```python
from build123d import *

# Parameters (mm, degrees)
F0_R     = 3
F1_DEPTH = 2
F2_T     = -1
F4_W     = 4
F4_H     = 1
F4_R     = 4
F4_R_2   = 3
F5_DEPTH = 1


# Not quite as in the source:
# - a feature of the source that left no trace in its solid (it failed there, or was rolled back) is left out


with BuildPart() as f1:
    # F0 (on Top) → F1 (new body)
    with BuildSketch(Plane.XY):
        with BuildLine():
            ThreePointArc((76, 31), (0, 107), (-76, 31))
            Line((-76, 31), (-76, -31))
            Line((-76, -31), (-76, -69))
            Line((-76, -69), (-70, -69))
            Line((-70, -69), (-70, -47.9877756238))
            Line((-70, -47.9877756238), (-66, -47.9877756238))
            Line((-66, -47.9877756238), (-66, -40.0317243588))
            ThreePointArc((-66, -40.0317243588), (-61.2993566139, -29.9422610746), (-70, -23.00020646))
            Line((-70, -23.00020646), (-70, 31))
            ThreePointArc((-70, 31), (-66.3741952073, 53.2365962005), (-55.8723939833, 73.1696050559))
            ThreePointArc((-55.8723939833, 73.1696050559), (-43.5714285714, 73.6911069456), (-43.3010754044, 86.0001533527))
            ThreePointArc((-43.3010754044, 86.0001533527), (-22.9127613494, 97.1438233499), (0, 101))
            ThreePointArc((0, 101), (22.9127613494, 97.1438233499), (43.3010754044, 86.0001533527))
            ThreePointArc((43.3010754044, 86.0001533527), (43.5714285714, 73.6911069456), (55.8723939833, 73.1696050559))
            ThreePointArc((55.8723939833, 73.1696050559), (66.3741952073, 53.2365962005), (70, 31))
            Line((70, 31), (70, -23.00020646))
            ThreePointArc((70, -23.00020646), (61.2993566139, -29.9422610746), (66, -40.0317243588))
            Line((66, -40.0317243588), (66, -47.9877756238))
            Line((66, -47.9877756238), (70, -47.9877756238))
            Line((70, -47.9877756238), (70, -69))
            Line((70, -69), (76, -69))
            Line((76, -69), (76, -31))
            Line((76, -31), (76, 31))
        make_face()
        with Locations((-70.0609609485, -32)):
            Circle(F0_R, mode=Mode.SUBTRACT)
        with Locations((70.0609609485, -32)):
            Circle(F0_R, mode=Mode.SUBTRACT)
        with Locations((-50, 79.9897948557)):
            Circle(F0_R, mode=Mode.SUBTRACT)
        with Locations((50, 79.9897948557)):
            Circle(F0_R, mode=Mode.SUBTRACT)
    extrude(amount=F1_DEPTH)

    # F2
    f2_openings = [f1.faces().sort_by_distance(p)[0] for p in [
        (0, 104.674489, 2),
    ]]
    offset(amount=F2_T, openings=f2_openings, kind=Kind.INTERSECTION)

    # F4 (on face) → F5 (cut)
    with BuildSketch(Plane.XY.offset(2)):
        with Locations((73, -68.5)):
            Rectangle(F4_W, F4_H)
        with Locations((-73, -68.5)):
            Rectangle(F4_W, F4_H)
        with Locations((-70.0609609485, -32)):
            Circle(F4_R)
        with Locations((-70.0609609485, -32)):
            Circle(F4_R_2, mode=Mode.SUBTRACT)
        with Locations((70.0609609485, -32)):
            Circle(F4_R)
        with Locations((70.0609609485, -32)):
            Circle(F4_R_2, mode=Mode.SUBTRACT)
        with Locations((-50, 79.9897948557)):
            Circle(F4_R)
        with Locations((-50, 79.9897948557)):
            Circle(F4_R_2, mode=Mode.SUBTRACT)
        with Locations((50, 79.9897948557)):
            Circle(F4_R)
        with Locations((50, 79.9897948557)):
            Circle(F4_R_2, mode=Mode.SUBTRACT)
    extrude(amount=-F5_DEPTH, mode=Mode.SUBTRACT)


solid = f1.part
```
Here's how the part is built. I have some questions about the finished solid (model axes, mm). A direction names the side the tool comes from. Round coordinates to 2 decimals unless told otherwise and drop trailing zeros. Order: outer loops, then holes, each group sorted by start corner. A loop starts at its lowest first (then second) coordinate and runs counter-clockwise, first axis right, second up. Notation, with made-up numbers: (83.5, 67) -> (111.5, 67) arc R22 ccw to (111.5, 92) -> close; hole circle Ø11 at (5.5, -33.75). An arc over 180 degrees is marked (long way). Use a Markdown table: item, result. Add a question column.
(1) For pin 1 Ø9.5 at (x, y) = (50, 79.99) entering from -Z; pin 2 Ø1.1 at (x, z) = (-68, 1.5) entering from +Y; pin 3 Ø1 at (x, z) = (31, 1.5) entering from +Y, each with a flat end and sliding along its axis, tell me the tip position at first contact or that it passes through.
(2) For faces 1 (the face through (61.34, -29.78, 0.99)), 2 (the face through (67.032, 54.404, 1.493)), which set-ups out of +Z, -Z, +X, -X, +Y, -Y let a thin tool reach every point of the face, with its end or its side?
(3) If we mould it in two halves opening along X, with no side actions, what happens to faces 3 (the face through (-72.44, -33.83, 0.49)), 4 (the face through (-51, 72, 0))? For each: released by +X, released by -X, zero draft, split by the parting line, or undercut.
(4) Suppose I cut it at D-D, the plane x = -29. Please give me the cut outline in (y, z), and give its area (3 significant figures).
(5) Suppose I cut it at A-A, the plane y = -32. Please give me the cut outline in (x, z), and give its area (3 significant figures).
(6) Suppose I cut it at C-C, the plane y = -7.5. Please give me the cut outline in (x, z), and give its area (3 significant figures).
(7) Suppose I cut it at B-B, the plane x = 50. Please give me the cut outline in (y, z), and give its area (3 significant figures).
(8) I need wall thicknesses on line 1 along X through (y, z) = (-51, 1.3); line 2 along X through (y, z) = (9.5, 0.9); line 3 along Y through (x, z) = (64, 1.6). Which ranges of each line are inside material? Lowest first, please.
Verdict:
| question | item | result |
|---|---|---|
| 1 | pin 1 | z = 0 |
| 1 | pin 2 | y = 66.02 |
| 1 | pin 3 | y = 100.61 |
| 2 | face 1 | +Z, -Z |
| 2 | face 2 | +Z |
| 3 | face 3 | undercut |
| 3 | face 4 | zero draft |
| 4 | outline | (94.71, 0) -> (101.25, 0) -> (101.25, 2) -> (100.17, 2) -> (100.17, 1) -> (95.81, 1) -> (95.81, 2) -> (94.71, 2) -> close |
| 4 | area | 8.72 mm2 |
| 5 | outline | (-76, 0) -> (-73.06, 0) -> (-73.06, 1) -> (-75, 1) -> (-75, 2) -> (-76, 2) -> close; (-67.06, 0) -> (-61.06, 0) -> (-61.06, 2) -> (-62.06, 2) -> (-62.06, 1) -> (-67.06, 1) -> close; (61.06, 0) -> (67.06, 0) -> (67.06, 1) -> (62.06, 1) -> (62.06, 2) -> (61.06, 2) -> close; (73.06, 0) -> (76, 0) -> (76, 2) -> (75, 2) -> (75, 1) -> (73.06, 1) -> close |
| 5 | area | 21.9 mm2 |
| 6 | outline | (-76, 0) -> (-70, 0) -> (-70, 2) -> (-71, 2) -> (-71, 1) -> (-75, 1) -> (-75, 2) -> (-76, 2) -> close; (70, 0) -> (76, 0) -> (76, 2) -> (75, 2) -> (75, 1) -> (71, 1) -> (71, 2) -> (70, 2) -> close |
| 6 | area | 16.0 mm2 |
| 7 | outline | (70.99, 0) -> (76.99, 0) -> (76.99, 1) -> (71.99, 1) -> (71.99, 2) -> (70.99, 2) -> close; (82.99, 0) -> (88.24, 0) -> (88.24, 2) -> (86.9, 2) -> (86.9, 1) -> (82.99, 1) -> close |
| 7 | area | 13.6 mm2 |
| 8 | line 1 | -76 to -75, -71 to -70, 70 to 71, 75 to 76 |
| 8 | line 2 | -76 to -70, 70 to 76 |
| 8 | line 3 | -38.65 to -37.22, -26.78 to -25.35, 59.35 to 61.74, 70.1 to 71.99 |
